Autodesk Inventor part; units mm, degrees
ref_plane "YZ Plane" through (0, 0, 0) normal (1, 0, 0) x (0, 1, 0)
ref_plane "XZ Plane" through (0, 0, 0) normal (0, 1, 0) x (-1, 0, 0)
ref_plane "XY Plane" through (0, 0, 0) normal (0, 0, 1) x (1, 0, 0)
sketch "Sketch1" plane through (0, 0, 0) normal (0, 1, 0) x (-1, 0, 0)
  point P0 (0, 0)
sketch "Sketch2" plane through (0, 0, 0) normal (0, 1, 0) x (-1, 0, 0)
  circle A0 centre (0, 0) radius 4.8
  dimension "d0" = 9.6
extrude "Extrusion1" add sketch "Sketch2" along normal blind 19
sketch "Sketch3" plane through (0, 19, 0) normal (0, 1, 0) x (1, 0, 0)
  circle A0 centre (0, 0) radius 3
  line L0 (-2.6263, 1.45) -> (2.6263, 1.45)
  circle A1 centre (0, 0) radius 3.15
  point P0 (0, 1.45)
  dimension "d3" = 6
  dimension "d4" = 1.45
  dimension "d13" = 6.3
sketch "shaft cutout" plane through (0, 0, 0) normal (0, -1, 0) x (1, 0, 0)
  circle A0 centre (0, 0) radius 3.075
  line L0 (2.7117, -1.45) -> (-2.7117, -1.45)
  point P0 (0, -1.45)
  point P1 (0, -1.45)
  dimension "d7" = 6.15
sketch "top spacer" plane through (0, 0, 0) normal (0, -1, 0) x (1, 0, 0)
  circle A0 centre (0, 0) radius 3.5
  dimension "d10" = 7
extrude "Extrusion6" cut sketch "shaft cutout" against normal blind 9 contours A0 L0 picked at (0.9722, -0.3362)
extrude "Extrusion7" cut sketch "top spacer" against normal blind 3
extrude "Extrusion8" add sketch "Sketch3" along normal blind 9 contours A0 L0 | L0 A0 | A1
properties part number "v6 Knob extender long_3DPrint"
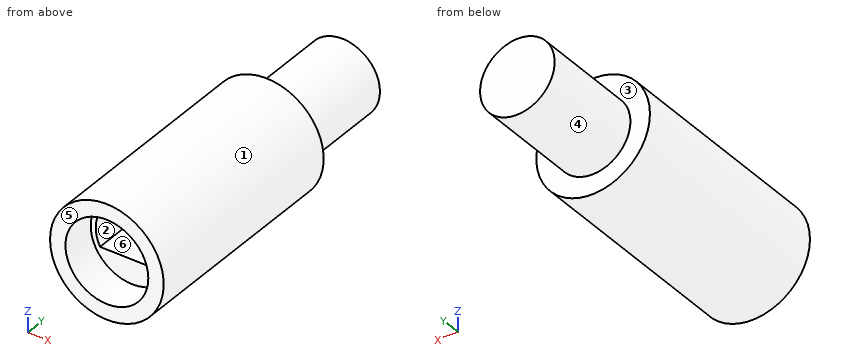
Model file for the job. Use its own axes, mm. Face numbers are marked on the shaded views. A direction names the side the tool comes from. Give positions to 0.01 mm unless a question says otherwise; leave off trailing zeros. Write each loop counter-clockwise with the first axis right and the second up, starting at its lowest first coordinate (ties: lowest second). Pieces come first, ordered by that corner, then holes. Notation, with made-up numbers: (83, 7.25) -> (97, 7.25) arc R11 cw to (97, 28.25) -> close; hole circle Ø10 at (19, 2.5). An arc over 180 degrees is marked (long way). Use CSV: the item, a comma, the result in double quotes. Start each with the question number.
1) Cut at B-B on x = 0. List the corners of the cut face in (y, z) (3 decimals), plus the area to 3 significant figures.
2) Two-plate mould, pull along X, no slides. Class the marked faces 4, 5 and 6: released by +X, released by -X, zero draft, split by the parting line, or undercut.
3) Tool access for the marked faces 1, 2 and 3: list every direction of +Z, -Z, +X, -X, +Y, -Y with a clear straight run to the whole face (end or side of a thin tool).
4) Pin check, flat tips, straight feed: P1, Ø2, axis at y = 22.5, z = 2.5, coming from the -X side; P2, Ø2, axis at x = -2.5, y = 21.5, coming from the +Z side; P3, Ø1, axis at y = 24.5, z = -1, coming from the -X side. Stop position of each tip, or through.
5) Cut at D-D on y = 25.75. List the corners of the cut face in (x, z), plus the area to 3 significant figures.
6) Cut at C-C on y = 2.25. List the corners of the cut face in (x, z), plus the area to 3 significant figures.
7) Cut at A-A on z = 0. List the corners of the cut face in (x, y) (3 decimals), plus the area to 3 significant figures.
8) Drill centre lines: L1, parallel to Z at x = 0, y = 2.15; L2, parallel to Y at x = -1.75, z = -2.25; L3, parallel to Z at x = 0, y = 7.5 (3 decimals). Where is each one in solid material? Low to high.
Final values:
1,outline,"(0, -4.8) -> (19, -4.8) -> (19, -3.15) -> (28, -3.15) -> (28, 3.15) -> (19, 3.15) -> (19, 4.8) -> (0, 4.8) -> (0, 3.5) -> (3, 3.5) -> (3, 3.075) -> (9, 3.075) -> (9, -1.45) -> (3, -1.45) -> (3, -3.5) -> (0, -3.5) -> close"
1,area,"191 mm2"
2,face 4,"split by the parting line"
2,face 5,"zero draft"
2,face 6,"undercut"
3,face 1,"+Y, -Y"
3,face 2,"-Y"
3,face 3,"+Y"
4,P1,"stops at x = -2.77"
4,P2,"stops at z = 2.77"
4,P3,"stops at x = -3.11"
5,outline,"circle Ø6.3 at (0, 0)"
5,area,"31.2 mm2"
6,outline,"circle Ø9.6 at (0, 0); hole circle Ø7 at (0, 0)"
6,area,"33.9 mm2"
7,outline,"(-4.8, 0) -> (-3.5, 0) -> (-3.5, 3) -> (-3.075, 3) -> (-3.075, 9) -> (3.075, 9) -> (3.075, 3) -> (3.5, 3) -> (3.5, 0) -> (4.8, 0) -> (4.8, 19) -> (3.15, 19) -> (3.15, 28) -> (-3.15, 28) -> (-3.15, 19) -> (-4.8, 19) -> close"
7,area,"181 mm2"
8,L1,"z = -4.8 to -3.5, 3.5 to 4.8"
8,L2,"y = 3 to 28"
8,L3,"z = -4.8 to -1.45, 3.075 to 4.8"
